Can you work these out from the model? Positions are in its coordinate system, mm. A direction names the side the tool comes from. Round coordinates to 2 decimals unless told otherwise and drop trailing zeros. Order: outer loops, then holes, each group sorted by start corner. A loop starts at its lowest first (then second) coordinate and runs counter-clockwise, first axis right, second up. Notation, with made-up numbers: M -19,85 L 2,85 A26 cw 2,124 Z; hole C 49,46.25 d10. An arc over 180 degrees is marked long. Answer as a JSON object with one key per item and string values. Group by question number.
```python
from build123d import *

# Parameters (mm, degrees)
F0_R     = 5
F0_R_2   = 2.9
F0_R_3   = 2.15
F1_DEPTH = 3
F2_DEPTH = 5
F3_R     = 2.9
F4_DEPTH = 3


with BuildPart() as f1:
    # F0 (on Top) → F1 (new body)
    with BuildSketch(Plane.XY):
        Circle(F0_R)
        Circle(F0_R_2, mode=Mode.SUBTRACT)
        Circle(F0_R_2)
        Circle(F0_R_3, mode=Mode.SUBTRACT)
    extrude(amount=F1_DEPTH)

    # F0 (on Top) → F2 (join)
    with BuildSketch(Plane.XY):
        Circle(F0_R_2)
        Circle(F0_R_3, mode=Mode.SUBTRACT)
    extrude(amount=-F2_DEPTH)

    # F3 (on face) → F4 (join)
    with BuildSketch(Plane(origin=(0, 0, -5), x_dir=(1, 0, 0), z_dir=(0, 0, -1))):
        Circle(F3_R)
    extrude(amount=F4_DEPTH)


solid = f1.part
```
1) I need wall thicknesses on line 1 along Y through (x, z) = (0, -1.75); line 2 along X through (y, z) = (-0.25, 1.25); line 3 along Z through (x, y) = (0.25, -4.5). Which ranges of each line are inside material? Lowest first, please.
2) We'd pull the mould along X, two halves only. Please class faces 1 (the face through (0, 0, -5)), 2 (the face through (1, -2.2, 3)), 3 (the face through (-1.08, -4.88, 1.48)): +X half, -X half, draft (parallel to the pull), parting line (faces both ways), or undercut.
3) If we section it at A-A on x = 0: Write out the boundary of the cut face in (y, z).
4) For pin 1 (2 mm diameter, centred on x = -3, z = -1.5, fed in from +Y); pin 2 (2 mm diameter, centred on x = 0.5, y = -0.5, fed in from +Z); pin 3 (3 mm diameter, centred on y = -3, z = -6.5, fed in from -X), each with a flat end and sliding along its axis, tell me the tip position at first contact or that it passes through.
5) Which directions (+Z, -Z, +X, -X, +Y, -Y) give clear straight access to the entire face, cutting with the end or side of a thin tool? Please do faces 4 (the face through (0, 0, -8)), 5 (the face through (-2.9, -0.1, -3.9)), 6 (the face through (-2.15, 0.09, -1.06)).
6) If we section it at C-C on z = 1.5: Write out the boundary of the cut face in (x, y).
7) If we section it at D-D on z = -4: Write out the boundary of the cut face in (x, y).
Findings:
{
 "1": {"line 1": "y = -2.9 to -2.15, 2.15 to 2.9", "line 2": "x = -4.99 to -2.14, 2.14 to 4.99", "line 3": "z = 0 to 3"},
 "2": {"face 1": "undercut", "face 2": "draft", "face 3": "parting line"},
 "3": {"outline": "M -5,0 L -2.9,0 L -2.9,-8 L 2.9,-8 L 2.9,0 L 5,0 L 5,3 L 2.15,3 L 2.15,-5 L -2.15,-5 L -2.15,3 L -5,3 Z"},
 "4": {"pin 1": "stops at y = 2.1", "pin 2": "stops at z = -5", "pin 3": "stops at x = -2.48"},
 "5": {"face 4": "-Z, +X, -X, +Y, -Y", "face 5": "-Z", "face 6": "+Z"},
 "6": {"outline": "C 0,0 d10; hole C 0,0 d4.3"},
 "7": {"outline": "C 0,0 d5.8; hole C 0,0 d4.3"}
}
